Verification items for the finished model (mm, model axes). Round coordinates to 2 decimals unless told otherwise and drop trailing zeros. Write each loop counter-clockwise with the first axis right and the second up, starting at its lowest first coordinate (ties: lowest second). Pieces come first, ordered by that corner, then holes. Notation, with made-up numbers: (65.5, 22.5) - (91.5, 22.5) arc R22 ccw to (91.5, 44.5) - close; hole circle Ø3 at (67, 79.5). An arc over 180 degrees is marked (long way). Answer as a JSON object with one key per item and string values. Group by question number.
1) Section check D-D (x = -13.8). Enter the section's corners in (y, z), then the cut area to 3 significant figures.
2) Go/stop test with flat-tipped pins: pin 1 Ø1.2 at (y, z) = (-23, 1.5) entering from -X; pin 2 Ø1.2 at (x, z) = (-23, 1.5) entering from +Y; pin 3 Ø0.7 at (y, z) = (24, 1.5) entering from +X. Record where each tip stops, or that it passes through.
3) Section check A-A (x = 0). Enter the section's corners in (y, z).
4) Section check C-C (z = 1.45). Enter the section's corners in (x, y).
5) Thickness scan on line 1 (X direction, y = -1.5, z = 1.65); line 2 (Y direction, x = 0, z = 0.95); line 3 (Y direction, x = 21.5, z = 0.2). Record the ranges inside material, lowest first.
6) Section check B-B (y = 0). Enter the section's corners in (x, z), then the cut area to 3 significant figures.
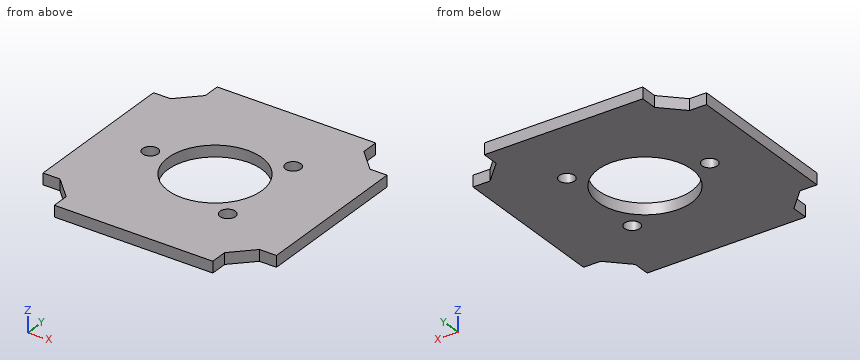
Autodesk Inventor part; units mm, degrees
ref_plane "Work Plane1" through (-29.1, -14.5, 2.4) normal (0, 0, -1) x (0, 1, 0)
ref_plane "YZ Plane" through (0, 0, 0) normal (1, 0, 0) x (0, 1, 0)
ref_plane "XZ Plane" through (0, 0, 0) normal (0, 1, 0) x (-1, 0, 0)
ref_plane "Work Plane1" through (-29.1, -14.5, 2.4) normal (0, 0, -1) x (0, 1, 0)
sketch "Sketch1" plane through (0, 0, 0) normal (0, 0, 1) x (1, 0, 0)
  line L0 (-34.86, 0) -> (34.86, 0) construction
  line L1 (0, -34.86) -> (0, 34.86) construction
  line L2 (0, 0) -> (11.1575, 11.1575) construction
  line L3 (0, 0) -> (15.7791, 0) construction
  line L4 (0, 24.9) -> (16.8009, 24.9)
  line L5 (16.8009, 24.9) -> (16.8009, 21.2415)
  line L6 (16.8009, 21.2415) -> (19.0212, 19.0212)
  line L7 (24.9, 0) -> (24.9, 16.8009)
  line L8 (24.9, 16.8009) -> (21.2415, 16.8009)
  line L9 (21.2415, 16.8009) -> (19.0212, 19.0212)
  line L10 (0, -24.9) -> (16.8009, -24.9)
  line L11 (16.8009, -24.9) -> (16.8009, -21.2415)
  line L12 (16.8009, -21.2415) -> (19.0212, -19.0212)
  line L13 (24.9, 0) -> (24.9, -16.8009)
  line L14 (24.9, -16.8009) -> (21.2415, -16.8009)
  line L15 (21.2415, -16.8009) -> (19.0212, -19.0212)
  line L16 (0, 24.9) -> (-16.8009, 24.9)
  line L17 (-16.8009, 24.9) -> (-16.8009, 21.2415)
  line L18 (-16.8009, 21.2415) -> (-19.0212, 19.0212)
  line L19 (-24.9, 16.8009) -> (-21.2415, 16.8009)
  line L20 (-21.2415, 16.8009) -> (-19.0212, 19.0212)
  line L21 (0, -24.9) -> (-16.8009, -24.9)
  line L22 (-16.8009, -24.9) -> (-16.8009, -21.2415)
  line L23 (-16.8009, -21.2415) -> (-19.0212, -19.0212)
  line L24 (-21.2415, -16.8009) -> (-19.0212, -19.0212)
  line L25 (-24.9, -16.8009) -> (-21.2415, -16.8009)
  line L26 (-24.9, 0) -> (-24.9, -16.8009)
  line L27 (-24.9, 0) -> (-24.9, 16.8009)
  circle A0 centre (0, 0) radius 10
  dimension "d0" = 45
  dimension "d2" = 24.9
  dimension "d3" = 3.14
  dimension "d4" = 26.9
  dimension "d5" = 20
extrude "Extrusion1" add sketch "Sketch1" along normal up to surface (2.4 mm away)
sketch "Sketch5" plane through (0, 0, 0) normal (0, 0, -1) x (-1, 0, 0)
  circle A0 centre (-9.7, 10) radius 1.4
  circle A1 centre (-9.7, -10) radius 1.4
  circle A2 centre (13.8, 0) radius 1.4
  point P0 (0, 0)
hole "Hole1" at (9.7, 10, 0) at (-13.8, 0, 0) at (9.7, -10, 0) direction (0, 0, 1) diameter 3.3 depth 12 tip angle 118
sketch "Skizze6" plane through (-16.8009, 24.9, 2.4) normal (0, 0, 1) x (1, 0, 0)
  circle A0 centre (3.0009, -24.9) radius 1.65 construction
  circle A1 centre (26.5009, -14.9) radius 1.65 construction
  circle A2 centre (26.5009, -34.9) radius 1.65 construction
  circle A3 centre (16.8009, -24.9) radius 10 construction
  line L0 (33.6017, -3.6585) -> (33.6017, 0)
  line L1 (33.6017, 0) -> (0, 0) construction
  line L2 (0, 0) -> (0, -3.6585)
  line L3 (0, -3.6585) -> (-4.4406, -8.0991)
  line L4 (-4.4406, -8.0991) -> (-8.0991, -8.0991)
  line L5 (-8.0991, -8.0991) -> (-8.0991, -41.7009) construction
  line L6 (-8.0991, -41.7009) -> (-4.4406, -41.7009)
  line L7 (-4.4406, -41.7009) -> (0, -46.1415)
  line L8 (0, -46.1415) -> (0, -49.8)
  line L9 (0, -49.8) -> (33.6017, -49.8) construction
  line L10 (33.6017, -49.8) -> (33.6017, -46.1415)
  line L11 (33.6017, -46.1415) -> (38.0423, -41.7009)
  line L12 (38.0423, -41.7009) -> (41.7009, -41.7009)
  line L13 (41.7009, -41.7009) -> (41.7009, -8.0991) construction
  line L14 (41.7009, -8.0991) -> (38.0423, -8.0991)
  line L15 (38.0423, -8.0991) -> (33.6017, -3.6585)
  line L16 (-0.1, 0.1) -> (33.7017, 0.1) construction
  line L17 (33.7017, 0.1) -> (33.7017, -3.6171)
  line L18 (33.7017, -3.6171) -> (38.0838, -7.9991)
  line L19 (38.0838, -7.9991) -> (41.8009, -7.9991)
  line L20 (41.8009, -7.9991) -> (41.8009, -41.8009) construction
  line L21 (41.8009, -41.8009) -> (38.0838, -41.8009)
  line L22 (38.0838, -41.8009) -> (33.7017, -46.1829)
  line L23 (33.7017, -46.1829) -> (33.7017, -49.9)
  line L24 (33.7017, -49.9) -> (-0.1, -49.9) construction
  line L25 (-0.1, -49.9) -> (-0.1, -46.1829)
  line L26 (-0.1, -46.1829) -> (-4.4821, -41.8009)
  line L27 (-4.4821, -41.8009) -> (-8.1991, -41.8009)
  line L28 (-8.1991, -41.8009) -> (-8.1991, -7.9991) construction
  line L29 (-8.1991, -7.9991) -> (-4.4821, -7.9991)
  line L30 (-4.4821, -7.9991) -> (-0.1, -3.6171)
  line L31 (-0.1, -3.6171) -> (-0.1, 0.1)
  line L32 (-8.0991, -8.0991) -> (-8.0991, -7.9991)
  line L33 (0, -3.6585) -> (0, 0)
  line L34 (0, 0) -> (-0.1, 0)
  line L35 (33.6017, 0) -> (33.6017, -3.6585)
  line L36 (33.6017, 0) -> (33.7017, 0)
  line L37 (41.7009, -8.0991) -> (41.7009, -7.9991)
  line L38 (41.7009, -41.7009) -> (41.7009, -8.0991)
  line L39 (41.7009, -41.7009) -> (41.7009, -41.8009)
  line L40 (33.6017, -49.8) -> (0, -49.8)
  line L41 (33.6017, -49.8) -> (33.7017, -49.8)
  line L42 (0, -49.8) -> (-0.1, -49.8)
  line L43 (-8.0991, -41.7009) -> (-8.0991, -41.8009)
  dimension "d25" = 0.1
extrude "IM_offset" add sketch "Skizze6" against normal up to surface (2.4 mm away)
properties part number "20_Cube_insert_Basler_acA1920_25gm_v3"
Returned:
{
 "1": {"outline": "(-24.9, 0) - (-1.65, 0) - (-1.65, 2.4) - (-24.9, 2.4) - close; (1.65, 0) - (24.9, 0) - (24.9, 2.4) - (1.65, 2.4) - close", "area": "112 mm2"},
 "2": {"pin 1": "x = -16.9", "pin 2": "y = 16.9", "pin 3": "x = 16.9"},
 "3": {"outline": "(-24.9, 0) - (-10, 0) - (-10, 2.4) - (-24.9, 2.4) - close; (10, 0) - (24.9, 0) - (24.9, 2.4) - (10, 2.4) - close"},
 "4": {"outline": "(-24.9, -16.9) - (-21.28, -16.9) - (-16.9, -21.28) - (-16.9, -24.9) - (16.9, -24.9) - (16.9, -21.28) - (21.28, -16.9) - (24.9, -16.9) - (24.9, 16.9) - (21.28, 16.9) - (16.9, 21.28) - (16.9, 24.9) - (-16.9, 24.9) - (-16.9, 21.28) - (-21.28, 16.9) - (-24.9, 16.9) - close; hole circle Ø3.3 at (-13.8, 0); hole circle Ø20 at (0, 0); hole circle Ø3.3 at (9.7, -10); hole circle Ø3.3 at (9.7, 10)"},
 "5": {"line 1": "-24.9 to -14.49, -13.11 to -9.89, 9.89 to 24.9", "line 2": "-24.9 to -10, 10 to 24.9", "line 3": "-16.9 to 16.9"},
 "6": {"outline": "(-24.9, 0) - (-15.45, 0) - (-15.45, 2.4) - (-24.9, 2.4) - close; (-12.15, 0) - (-10, 0) - (-10, 2.4) - (-12.15, 2.4) - close; (10, 0) - (24.9, 0) - (24.9, 2.4) - (10, 2.4) - close", "area": "63.6 mm2"}
}
